Geometry: final body of the model. Coordinates: model frame, mm. A direction names the side the tool comes from. Coordinates: 2 decimals unless noted, no trailing zeros. Write each loop counter-clockwise with the first axis right and the second up, starting at its lowest first coordinate (ties: lowest second). Pieces come first, ordered by that corner, then holes. Notation, with made-up numbers: (-12.75, -37) -> (-4.75, -37) arc R32 ccw to (-4.75, 2) -> close; hole circle Ø7 at (64.5, 21.5). An arc over 180 degrees is marked (long way). Answer as a JSON object with one key per item and string values. Group by question number.
```python
from build123d import *

# Parameters (mm, degrees)
SKETCH1_W           = 83.185
SKETCH1_H           = 59.69
BOSS_EXTRUDE1_DEPTH = 3.175
SKETCH2_W           = 16.637
SKETCH2_H           = 3.175
CUT_EXTRUDE1_DEPTH  = 3.175
LPATTERN1_COUNT     = 3
LPATTERN1_PITCH     = 33.274
SKETCH3_W           = 3.175
SKETCH3_H           = 11.938
CUT_EXTRUDE2_DEPTH  = 3.175
LPATTERN4_COUNT     = 3
LPATTERN4_PITCH     = 23.876


with BuildPart() as part:
    # Sketch1 → Boss-Extrude1 (new body)
    with BuildSketch(Plane(origin=(0, 0, 0), x_dir=(1, 0, 0), z_dir=(0, 1, 0))):
        Rectangle(SKETCH1_W, SKETCH1_H)
    extrude(amount=BOSS_EXTRUDE1_DEPTH)

    # Sketch2 → Cut-Extrude1 (cut)
    with BuildSketch(Plane(origin=(0, 3.175, 0), x_dir=(1, 0, 0), z_dir=(0, 1, 0))):
        with Locations((-33.274, 28.2575)):
            Rectangle(SKETCH2_W, SKETCH2_H)
        with Locations((-33.274, -28.2575)):
            Rectangle(SKETCH2_W, SKETCH2_H)
    cut_extrude1 = extrude(amount=-CUT_EXTRUDE1_DEPTH, mode=Mode.SUBTRACT)

    # LPattern1: Cut-Extrude1 ×3
    with Locations(*[(i * LPATTERN1_PITCH, 0, 0) for i in range(1, LPATTERN1_COUNT)]):
        add(cut_extrude1, mode=Mode.SUBTRACT)

    # Sketch3 → Cut-Extrude2 (cut)
    with BuildSketch(Plane(origin=(0, 3.175, 0), x_dir=(1, 0, 0), z_dir=(0, 1, 0))):
        with Locations((-40.005, 23.876)):
            Rectangle(SKETCH3_W, SKETCH3_H)
        with Locations((40.005, 23.876)):
            Rectangle(SKETCH3_W, SKETCH3_H)
    cut_extrude2 = extrude(amount=-CUT_EXTRUDE2_DEPTH, mode=Mode.SUBTRACT)

    # LPattern4: Cut-Extrude2 ×3
    with Locations(*[(0, 0, i * LPATTERN4_PITCH) for i in range(1, LPATTERN4_COUNT)]):
        add(cut_extrude2, mode=Mode.SUBTRACT)


solid = part.part
```
Item 1: Contact query for flat-ended pins moving along their axis: pin 1 (1.6 mm diameter, centred on x = -35, y = 1.5, fed in from +Z); pin 2 (1.6 mm diameter, centred on y = 2, z = -28.5, fed in from +X); pin 3 (1.5 mm diameter, centred on y = 2.5, z = 23, fed in from +X). Output: stop coordinate, or through.
Item 2: Ray query, L1, parallel to Z at x = 7, y = 0.85; L2, parallel to X at y = 1.65, z = 25. Return the intervals inside material, ascending. Write a range as [from, to].
Item 3: Section A-A on z = -2. Output: boundary loops of the cut face in (x, y) (1 decimal), then the cut area to 3 significant figures.
Item 4: Set-up query: faces 4 (the flat face through (38.418, 2, 22)), 5 (the flat face through (8.318, 2, 28)), 6 (the flat face through (-8.318, 2, -28)), 7 (the flat face through (-40, 2, -17.907)). Return all of +Z, -Z, +X, -X, +Y, -Y with unobstructed straight access to the full face (end or side cutting, diameter ignored); none if empty.
Item 5: Mould query, pull axis X, two halves, no side actions, for faces 1 (the flat face through (0, 2, 26.67)), 2 (the flat face through (-38.418, 2, 22)), 3 (the flat face through (41.592, 2, -12)). Classes: +X half, -X half, draft (parallel to the pull), parting line (faces both ways), or undercut.
Item 6: Section B-B on x = 35.5. Output: boundary loops of the cut face in (y, z) (3 decimals), then the cut area to 3 significant figures.
Answer sheet:
{
 "1": {"pin 1": "stops at z = 26.67", "pin 2": "stops at x = 24.96", "pin 3": "stops at x = 38.42"},
 "2": {"L1": "z = [-26.67, 26.67]", "L2": "x = [-38.42, 38.42]"},
 "3": {"outline": "(-38.4, 0) -> (38.4, 0) -> (38.4, 3.2) -> (-38.4, 3.2) -> close", "area": "244 mm^2"},
 "4": {"face 4": "+Z, +X, +Y, -Y", "face 5": "+Z, +Y, -Y", "face 6": "-Z, +Y, -Y", "face 7": "-Z, -X, +Y, -Y"},
 "5": {"face 1": "undercut", "face 2": "-X half", "face 3": "+X half"},
 "6": {"outline": "(0, -26.67) -> (3.175, -26.67) -> (3.175, 26.67) -> (0, 26.67) -> close", "area": "169 mm^2"}
}
